Part model, mm, in its own coordinate system. Give positions to 0.01 mm unless a question says otherwise; leave off trailing zeros. Order: outer loops, then holes, each group sorted by start corner. A loop starts at its lowest first (then second) coordinate and runs counter-clockwise, first axis right, second up. Notation, with made-up numbers: (89, 68) -> (112, 68) arc R16 cw to (112, 77) -> close; hole circle Ø2 at (-12, -12.75). An arc over 180 degrees is marked (long way). Write item = value, one per line. Start each with the question number.
Item 1: Band-saw the part on A-A on x = 112.5. Write the cut outline in (y, z).
Item 2: Flat gauge pins, fed straight in: P1, Ø5, axis at x = 150, y = -30, coming from the -Z side; P2, Ø3.5, axis at x = 0, y = 30, coming from the -Z side; P3, Ø2.5, axis at x = 30, y = -30, coming from the -Z side; P4, Ø0.9, axis at y = 25, z = -0.5, coming from the -X side. Where does each tip first touch, or does it go through?
Item 3: Drill centre lines: line 1 along Y through (x, z) = (145.4, 0); line 2 along Z through (x, y) = (145.8, 24.5); line 3 along Y through (x, z) = (150, 0.9). Where is each one in solid material? Low to high.
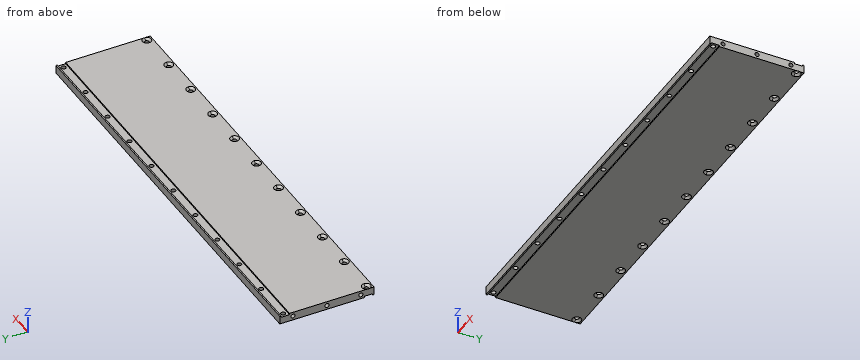
```python
from build123d import *

# Parameters (mm, degrees)
SKETCH_1_W                     = 306
SKETCH_1_H                     = 68
EXTRUDE_1_DEPTH                = 3
CUT_EXTRUDE_START              = 3
SKETCH_1_3_W                   = 306
SKETCH_1_3_H                   = 6
CUT_EXTRUDE_1_DEPTH            = 1
CUT_EXTRUDE_START_2            = -3
SKETCH_1_4_W                   = 306
SKETCH_1_4_H                   = 6
CUT_EXTRUDE_2_DEPTH            = 1
HOLE_START                     = -4
HOLE_WIZARD_M3_1_OUTLINE_R     = 1.6
HOLE_WIZARD_M3_1_DEPTH         = 8
M3X0_5_1_D                     = 2.5
M3X0_5_1_DEPTH                 = 8.5
M3X0_5_1_CBORE_D               = 3
M3X0_5_1_CBORE_DEPTH           = 6
M3X0_5_1_TIP                   = 0.751075774
M3X0_5_1_ON_FACE_2_D           = 2.5
M3X0_5_1_ON_FACE_2_DEPTH       = 8.5
M3X0_5_1_ON_FACE_2_CBORE_D     = 3
M3X0_5_1_ON_FACE_2_CBORE_DEPTH = 6
M3X0_5_1_ON_FACE_2_TIP         = 0.751075774
PATTERN_LINEAR_1_COUNT         = 11
PATTERN_LINEAR_1_PITCH         = 30


with BuildPart() as part:
    # ｽｹｯﾁ1 → ﾎﾞｽ - 押し出し1 (new, symmetric)
    with BuildSketch(Plane.XY):
        Rectangle(SKETCH_1_W, SKETCH_1_H)
    extrude(amount=EXTRUDE_1_DEPTH, both=True)

    # ｽｹｯﾁ1<3> → ｶｯﾄ - 押し出し1 (cut)
    with BuildSketch(Plane.XY.offset(CUT_EXTRUDE_START)):
        with Locations((0, 30)):
            Rectangle(SKETCH_1_3_W, SKETCH_1_3_H)
    extrude(amount=-CUT_EXTRUDE_1_DEPTH, mode=Mode.SUBTRACT)

    # ｽｹｯﾁ1<4> → ｶｯﾄ - 押し出し2 (cut)
    with BuildSketch(Plane.XY.offset(CUT_EXTRUDE_START_2)):
        with Locations((0, -30)):
            Rectangle(SKETCH_1_4_W, SKETCH_1_4_H)
    extrude(amount=CUT_EXTRUDE_2_DEPTH, mode=Mode.SUBTRACT)

    # M3 丸皿ねじ用皿穴1: read off the stored shape, not the designer's step
    # M3 丸皿ねじ用皿穴1 outline → M3 丸皿ねじ用皿穴1 (cut)
    with BuildSketch(Plane.XY.offset(HOLE_START)):
        with Locations((-150, -30)):
            Circle(HOLE_WIZARD_M3_1_OUTLINE_R)
        with Locations((-150, 30)):
            Circle(HOLE_WIZARD_M3_1_OUTLINE_R)
    hole_wizard_m3_1 = extrude(amount=HOLE_WIZARD_M3_1_DEPTH, mode=Mode.SUBTRACT)

    # Hole Wizard M3 _1 2: loft between two sections, ruled curve by curve
    hole_wizard_m3_1_2_from = [
        Edge.make_three_point_arc((-148.4, -30, 1.45), (-150, -28.4, 1.45), (-151.6, -30, 1.45)),
        Edge.make_three_point_arc((-151.6, -30, 1.45), (-150, -31.6, 1.45), (-148.4, -30, 1.45)),
    ]
    hole_wizard_m3_1_2_to = [
        Edge.make_three_point_arc((-146.849999512, -30, 3.000000488), (-150, -26.849999512, 3.000000488), (-153.150000488, -30, 3.000000488)),
        Edge.make_three_point_arc((-153.150000488, -30, 3.000000488), (-150, -33.150000488, 3.000000488), (-146.849999512, -30, 3.000000488)),
    ]
    hole_wizard_m3_1_2 = Solid(Shell([*[Face.make_surface_from_curves(hole_wizard_m3_1_2_from[k], hole_wizard_m3_1_2_to[k]) for k in range(2)], Face(Wire(hole_wizard_m3_1_2_from)), Face(Wire(hole_wizard_m3_1_2_to))]))
    add(hole_wizard_m3_1_2, mode=Mode.SUBTRACT)

    # Hole Wizard M3 _1 3: loft between two sections, ruled curve by curve
    hole_wizard_m3_1_3_from = [
        Edge.make_three_point_arc((-151.6, 30, -1.45), (-150, 31.6, -1.45), (-148.4, 30, -1.45)),
        Edge.make_three_point_arc((-148.4, 30, -1.45), (-150, 28.4, -1.45), (-151.6, 30, -1.45)),
    ]
    hole_wizard_m3_1_3_to = [
        Edge.make_three_point_arc((-153.150000488, 30, -3.000000488), (-150, 33.150000488, -3.000000488), (-146.849999512, 30, -3.000000488)),
        Edge.make_three_point_arc((-146.849999512, 30, -3.000000488), (-150, 26.849999512, -3.000000488), (-153.150000488, 30, -3.000000488)),
    ]
    hole_wizard_m3_1_3 = Solid(Shell([*[Face.make_surface_from_curves(hole_wizard_m3_1_3_from[k], hole_wizard_m3_1_3_to[k]) for k in range(2)], Face(Wire(hole_wizard_m3_1_3_from)), Face(Wire(hole_wizard_m3_1_3_to))]))
    add(hole_wizard_m3_1_3, mode=Mode.SUBTRACT)

    # M3x0.5 ねじ穴1
    with Locations(Plane(origin=(-153, 24.5, 0), x_dir=(0, 0, -1), z_dir=(-1, 0, 0))):
        with Locations((0, 0), (0, 49), (0, 24.5)):
            CounterBoreHole(M3X0_5_1_D / 2, M3X0_5_1_CBORE_D / 2, M3X0_5_1_CBORE_DEPTH, depth=M3X0_5_1_DEPTH)
            with Locations((0, 0, -(M3X0_5_1_DEPTH + M3X0_5_1_TIP / 2))):  # 118° drill point
                Cone(0, M3X0_5_1_D / 2, M3X0_5_1_TIP, mode=Mode.SUBTRACT)

    # M3x0.5 ねじ穴1 on face 2
    with Locations(Plane(origin=(153, 24.5, 0), x_dir=(0, 0, 1), z_dir=(1, 0, 0))):
        with Locations((0, 0), (0, 49), (0, 24.5)):
            CounterBoreHole(M3X0_5_1_ON_FACE_2_D / 2, M3X0_5_1_ON_FACE_2_CBORE_D / 2, M3X0_5_1_ON_FACE_2_CBORE_DEPTH, depth=M3X0_5_1_ON_FACE_2_DEPTH)
            with Locations((0, 0, -(M3X0_5_1_ON_FACE_2_DEPTH + M3X0_5_1_ON_FACE_2_TIP / 2))):  # 118° drill point
                Cone(0, M3X0_5_1_ON_FACE_2_D / 2, M3X0_5_1_ON_FACE_2_TIP, mode=Mode.SUBTRACT)

    # 直線ﾊﾟﾀｰﾝ1: M3 丸皿ねじ用皿穴1, Hole Wizard M3 _1 2, Hole Wizard M3 _1 3 ×11
    with Locations(*[(i * PATTERN_LINEAR_1_PITCH, 0, 0) for i in range(1, PATTERN_LINEAR_1_COUNT)]):
        add(hole_wizard_m3_1, mode=Mode.SUBTRACT)
        add(hole_wizard_m3_1_2, mode=Mode.SUBTRACT)
        add(hole_wizard_m3_1_3, mode=Mode.SUBTRACT)


solid = part.part
```
Values found:
q1.outline = (-34, -3) -> (-33, -3) -> (-33, -2) -> (-27, -2) -> (-27, -3) -> (34, -3) -> (34, 3) -> (33, 3) -> (33, 2) -> (27, 2) -> (27, 3) -> (-34, 3) -> close
q2.P1 = -2
q2.P2 = -1.6
q2.P3 = through
q2.P4 = -144.44
q3.line_1 = -34 to -25.75, -23.25 to -1.25, 1.25 to 23.25, 25.75 to 34
q3.line_2 = -3 to -1.25, 1.25 to 3
q3.line_3 = -34 to -31.6, -28.4 to -25.7, -23.3 to -1.2, 1.2 to 23.3, 25.7 to 28.4, 31.6 to 34
